Autodesk Inventor part; units mm, degrees
ref_plane "YZ Plane" through (0, 0, 0) normal (1, 0, 0) x (0, 1, 0)
ref_plane "XZ Plane" through (0, 0, 0) normal (0, 1, 0) x (-1, 0, 0)
ref_plane "XY Plane" through (0, 0, 0) normal (0, 0, 1) x (1, 0, 0)
sketch "Sketch1" plane through (0, 0, 0) normal (0, 0, 1) x (1, 0, 0)
  line L0 (48.7872, 31.5555) -> (48.7872, -28.4445)
  line L1 (13.7872, 31.5555) -> (13.7872, -28.4445)
  arc A0 (13.7872, -28.4445) -> (-11.2128, -71.7458) centre (76.1621, -93.3242) ccw
  line L2 (13.7872, -28.4445) -> (-11.2128, -71.7458) construction
  line L3 (13.7872, -28.4445) -> (63.7872, -28.4445) construction
  line L4 (-11.2128, -71.7458) -> (-11.2128, -121.7458)
  arc A1 (73.6491, -71.1938) -> (48.7872, -28.4445) centre (-13.5876, -93.3242) ccw
  line L5 (73.6491, -71.1938) -> (73.6491, -121.1332)
  line L6 (23.7872, -121.7458) -> (23.7872, -76.5352)
  arc A2 (31.2872, -61.5241) -> (23.7872, -76.5352) centre (76.1621, -93.3242) ccw
  arc A3 (38.6491, -76.1101) -> (31.2872, -61.5241) centre (-13.5876, -93.3242) ccw
  line L7 (38.6491, -76.1101) -> (38.6491, -121.1332)
  line L8 (-18.7128, -121.1332) -> (-18.7128, -70.8519)
  arc A4 (6.2872, -25.326) -> (-18.7128, -70.8519) centre (76.1621, -93.3242) ccw
  line L9 (6.2872, -25.326) -> (6.2872, 37.168)
  line L10 (6.2872, 37.168) -> (56.2872, 37.168)
  line L11 (56.2872, 37.168) -> (56.2872, -25.326)
  arc A5 (81.2182, -70.5622) -> (56.2872, -25.326) centre (-13.5876, -93.3242) ccw
  line L12 (81.2182, -70.5622) -> (81.2182, -121.1332)
  line L13 (-18.7128, -121.1332) -> (81.2182, -121.1332)
  line L14 (13.7872, 31.5555) -> (13.7872, 37.168)
  line L15 (48.7872, 31.5555) -> (48.7872, 37.168)
  line L16 (33.6491, -121.1332) -> (33.6491, -85.5895)
  line L17 (28.7872, -85.5895) -> (28.7872, -121.7458)
  line L18 (23.7872, -85.5895) -> (28.7872, -85.5895)
  line L19 (33.6491, -85.5895) -> (38.6491, -85.5895)
  line L20 (48.4283, 31.5555) -> (48.7872, 31.5555)
  line L21 (13.7872, 2.168) -> (13.7872, 22.168)
  line L22 (48.7872, 2.168) -> (48.7872, 22.168)
  line L23 (73.6491, -101.1332) -> (73.6491, -81.1332)
  line L24 (-11.2128, -81.1332) -> (-11.2128, -101.1332)
  line L25 (79.0378, -80.1332) -> (84.0378, -80.1332)
  line L26 (84.0378, -80.1332) -> (84.0378, -101.1332)
  line L27 (48.7872, 1.168) -> (48.7872, 22.168)
  line L28 (8.7872, 22.168) -> (13.7872, 22.168)
  line L29 (13.7872, 22.168) -> (13.7872, 1.168)
  line L30 (13.7872, 1.168) -> (8.7872, 1.168)
  line L31 (8.7872, 1.168) -> (8.7872, 22.168)
  line L32 (48.7872, 22.168) -> (53.7877, 22.168)
  line L33 (53.7877, 22.168) -> (53.7877, 2.168)
  line L34 (53.7877, 2.168) -> (48.7872, 2.168)
  line L35 (48.7872, 2.168) -> (48.7872, 22.168)
  line L36 (21.7872, 37.168) -> (16.2872, 27.6417)
  line L37 (21.7872, 37.168) -> (32.7872, 37.168) construction
  line L38 (16.2872, 27.6417) -> (47.2872, 27.6417)
  line L39 (47.2872, 27.6417) -> (41.7872, 37.168)
  line L40 (-11.2128, -81.1332) -> (-16.2128, -81.1332)
  line L41 (-16.2128, -81.1332) -> (-16.2128, -101.1332)
  line L42 (-16.2128, -101.1332) -> (-11.2128, -101.1332)
  line L43 (-11.2128, -101.1332) -> (-11.2128, -81.1332)
  line L44 (73.6491, -81.1332) -> (78.6491, -81.1332)
  line L45 (78.6491, -81.1332) -> (78.6491, -101.1332)
  line L46 (78.6491, -101.1332) -> (73.6491, -101.1332)
  line L47 (73.6491, -101.1332) -> (73.6491, -81.1332)
  point P0 (0, 0)
  point P1 (-11.2128, -121.1332)
  point P2 (23.7872, -121.1332)
  point P3 (36.2872, -121.7458)
  point P4 (71.2872, -121.7458)
  point P5 (28.7872, -121.1332)
  point P6 (31.2872, -121.7458)
  point P7 (81.2182, -80.1332)
  point P8 (13.7872, 22.168)
  point P9 (13.7872, 1.168)
  point P10 (48.7872, 2.168)
  point P11 (48.7872, 22.168)
  dimension "d0" = 35
  dimension "d1" = 60
  dimension "d2" = 50
  dimension "d3" = 120
  dimension "d4" = 90
  dimension "d5" = 50
  dimension "d6" = 35
  dimension "d7" = 7.5
  dimension "d12" = 5
  dimension "d16" = 7.5
  dimension "d22" = 158.3013
  dimension "d29" = 0
  dimension "d31" = 21
  dimension "d36" = 5
  dimension "d37" = 21
  dimension "d39" = 15
  dimension "d44" = 2.5
  dimension "d45" = 15
  dimension "d46" = 5.0004
  dimension "d47" = 20
  dimension "d48" = 90
  dimension "d49" = 90
  dimension "d50" = 2.8196
  dimension "d51" = 10.3887
  dimension "d52" = 27.7505
  dimension "d53" = 30.2501
  dimension "d54" = 45.3887
  dimension "d55" = 55.2505
  dimension "d58" = 111.6887
  dimension "d59" = 51.6887
  dimension "d60" = 5.4563
  dimension "d61" = 84.0378
  dimension "d62" = 80.1333
  dimension "d63" = 9.571
  dimension "d64" = 1
  dimension "d66" = 12.7505
  dimension "d67" = 41.6125
  dimension "d68" = 102.3013
  dimension "d69" = 82.3013
  dimension "d70" = 81.3013
  dimension "d71" = 47.7505
  dimension "d72" = 41.6125
  dimension "d73" = 52.7505
  dimension "d74" = 41.6125
  dimension "d75" = 55.2505
  dimension "d76" = 41
  dimension "d77" = 41.6125
  dimension "d78" = 60.2505
  dimension "d79" = 41
  dimension "d80" = 41.6125
  dimension "d81" = 102.3013
  dimension "d82" = 82.3013
  dimension "d83" = 1
  dimension "d84" = 21
  dimension "d85" = 95.2505
  dimension "d86" = 41
  dimension "d87" = 11
  dimension "d88" = 120
  dimension "d89" = 31
  dimension "d90" = 11
  dimension "d91" = 60
  dimension "d92" = 14.5
  dimension "d93" = 5
  dimension "d94" = 20
extrude "Extrusion1" add sketch "Sketch1" along normal blind 5 contours L15 L10 L11 A5 L12 L13 L5 L46 L45 L44 A1 L0 L34 L33 L32 | L0 A1 L5 L13 L7 A3 A2 L6 L4 A0 L1 L14 L10 L36 L38 L39 L15 | L14 L1 L28 L31 L30 A0 L4 L40 L41 L42 L13 L8 A4 L9 L10
sketch "Sketch2" plane through (0, 0, 5) normal (0, 0, 1) x (1, 0, 0)
  circle A0 centre (57.4252, -84.5438) radius 3
  circle A1 centre (5.4252, -84.5438) radius 3
  point P0 (0, 0)
  dimension "d99" = 6
  dimension "d100" = 6
  dimension "d101" = 52
extrude "Extrusion3" cut sketch "Sketch2" against normal blind 5
equation "\"d16\" = d7"
properties part number "newmiddle"
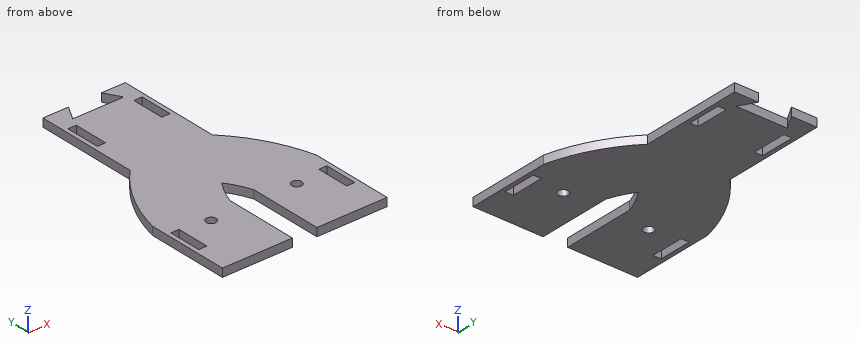
Verification items for the finished model (mm, model axes). Coordinates: 2 decimals unless noted, no trailing zeros. Order: outer loops, then holes, each group sorted by start corner. A loop starts at its lowest first (then second) coordinate and runs counter-clockwise, first axis right, second up. Notation, with made-up numbers: (-20.75, -13.5) - (-0.75, -13.5) arc R23 cw to (-0.75, 21.5) - close; hole circle Ø1 at (75.25, 23). An arc over 180 degrees is marked (long way). Return JSON: item names as keys, results as strings.
(1) Section check A-A, the plane y = -93. Record the cut outline in (x, z).
Filled sheet:
{"outline": "(-18.71, 0) - (-16.21, 0) - (-16.21, 5) - (-18.71, 5) - close; (-11.21, 0) - (23.79, 0) - (23.79, 5) - (-11.21, 5) - close; (38.65, 0) - (73.65, 0) - (73.65, 5) - (38.65, 5) - close; (78.65, 0) - (81.22, 0) - (81.22, 5) - (78.65, 5) - close"}
(2) Section check C-C, the plane x = 4. Record the cut outline in (y, z).
Filled sheet:
{"outline": "(-121.13, 0) - (-87.18, 0) - (-87.18, 5) - (-121.13, 5) - close; (-81.9, 0) - (-27.76, 0) - (-27.76, 5) - (-81.9, 5) - close"}
(3) Section check B-B, the plane y = -111. Record the cut outline in (x, z), and give its area (3 significant figures).
Filled sheet:
{"outline": "(-18.71, 0) - (23.79, 0) - (23.79, 5) - (-18.71, 5) - close; (38.65, 0) - (81.22, 0) - (81.22, 5) - (38.65, 5) - close", "area": "425 mm^2"}
(4) Thickness scan on line 1 along X through (y, z) = (9, 2.2); line 2 along X through (y, z) = (-94, 2.65); line 3 along X through (y, z) = (-81, 1). Record the ranges inside material, lowest first.
Filled sheet:
{"line 1": "x = 6.29 to 8.79, 13.79 to 48.79, 53.79 to 56.29", "line 2": "x = -18.71 to -16.21, -11.21 to 23.79, 38.65 to 73.65, 78.65 to 81.22", "line 3": "x = -18.71 to 23.79, 38.65 to 81.22"}
(5) Go/stop test with flat-tipped pins: pin 1 (1.5 mm diameter, centred on y = 17, z = 2.5, fed in from -X); pin 2 (1.5 mm diameter, centred on y = 14.5, z = 2.5, fed in from +X); pin 3 (2 mm diameter, centred on y = -31.5, z = 3.5, fed in from -X). Record where each tip stops, or that it passes through.
Filled sheet:
{"pin 1": "stops at x = 6.29", "pin 2": "stops at x = 56.29", "pin 3": "stops at x = -0.04"}
(6) Section check D-D, the plane z = 3.35. Give the number of separate pieces and of enclosed holes in the cut face, and give its area (3 significant figures).
Filled sheet:
{"separate pieces": "1", "enclosed holes": "6", "area": "10,300 mm^2"}
